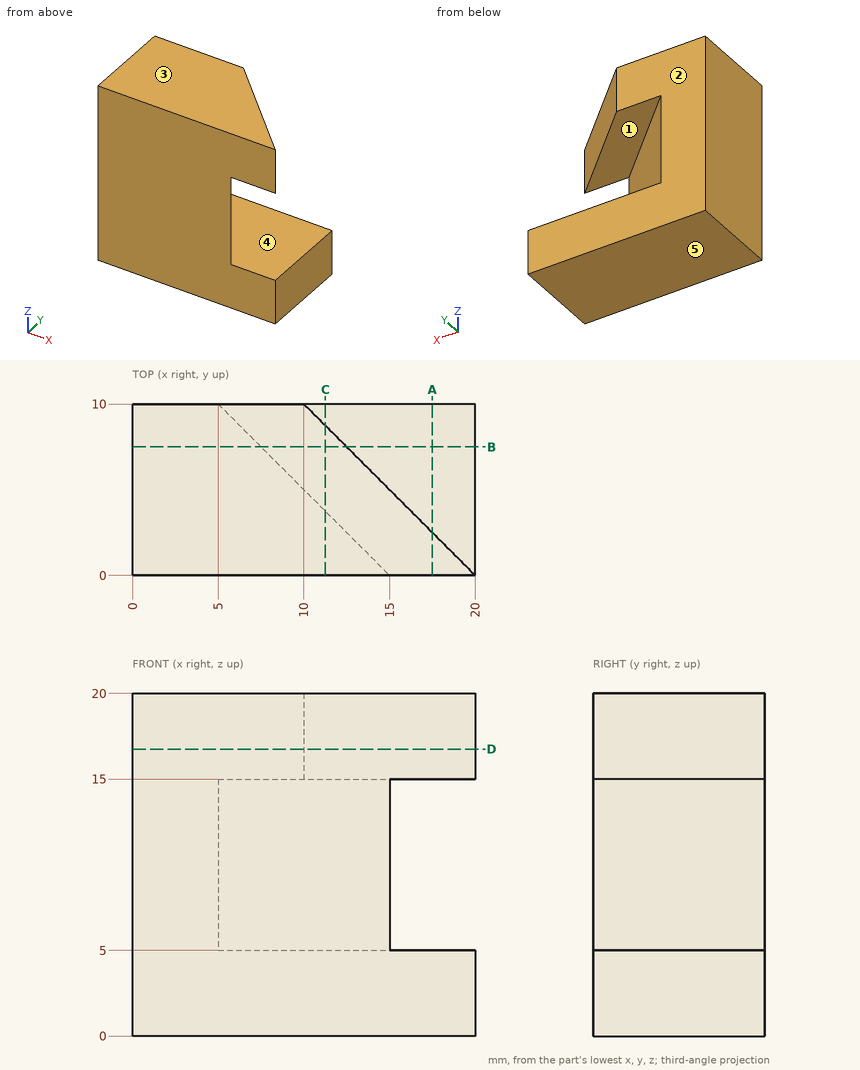
Geometry: see drawing. Coordinates: mm, zero at the bounding-box minimum. A direction names the side the tool comes from. Coordinates: 2 decimals unless noted, no trailing zeros. Order: outer loops, then holes, each group sorted by start corner. A loop starts at its lowest first (then second) coordinate and runs counter-clockwise, first axis right, second up. Notation, with made-up numbers: M 72.25,-15 L 78.25,-15 A31 cw 78.25,21 Z; hole C 18.25,26 d4. An arc over 180 degrees is marked long. Answer as CSV lines item,"result".
1. Section B-B (y = 7.5). Return the cut outline in (x, z).
Reported:
outline,"M 0,0 L 20,0 L 20,5 L 7.5,5 L 7.5,15 L 12.5,15 L 12.5,20 L 0,20 Z"
2. Section A-A (x = 17.5). Return the cut outline in (y, z).
Reported:
outline,"M 0,0 L 10,0 L 10,5 L 0,5 Z; M 0,15 L 2.5,15 L 2.5,20 L 0,20 Z"
3. Pull-direction query (Z, two-part tool) for the marked faces 1, 2 and 3; classes: released by +Z, released by -Z, zero draft, split by the parting line, or undercut.
Reported:
face 1,"undercut"
face 2,"zero draft"
face 3,"released by +Z"
4. Section D-D (z = 16.75). Return the cut outline in (x, y), then the cut area to 3 significant figures.
Reported:
outline,"M 0,0 L 20,0 L 10,10 L 0,10 Z"
area,"150 mm2"
5. Access query for the marked faces 4 and 5. Directions: +Z, -Z, +X, -X, +Y, -Y. A direction counts if a zero-diameter tool reaches every point of the face in a straight line with its end or side. Return the directions, or none.
Reported:
face 4,"+X, +Y"
face 5,"-Z, +X, -X, +Y, -Y"
6. Section C-C (x = 11.25). Return the cut outline in (y, z), then the cut area to 3 significant figures.
Reported:
outline,"M 0,0 L 10,0 L 10,5 L 3.75,5 L 3.75,15 L 8.75,15 L 8.75,20 L 0,20 Z"
area,"131 mm2"
7. Material intervals for line 1 (Z direction, x = 16, y = 6); line 2 (X direction, y = 5.5, z = 12.75), sorted ascending. Write a range as from..to.
Reported:
line 1,"0..5"
line 2,"0..9.5"
